Here's how the part is built. I have some questions about the finished solid (model axes, mm). A direction names the side the tool comes from. Round coordinates to 2 decimals unless told otherwise and drop trailing zeros. Loops run counter-clockwise (first coordinate to the right, second up) from the corner with the lowest first, then second, coordinate; pieces in that order, holes last. Notation, with made-up numbers: M -21.75,67.25 L -3.75,67.25 A9 cw -3.75,71.25 Z; hole C -26.5,22.25 d4. An arc over 180 degrees is marked long. Use a Markdown table: item, result.
```python
from build123d import *

# Parameters (mm, degrees)
SKETCH2_R           = 4
BOSS_EXTRUDE1_DEPTH = 25
CUT_EXTRUDE1_DEPTH  = 7
SKETCH6_W           = 0.80480735
SKETCH6_H           = 0.88864145
SKETCH6_W_2         = 0.905408268
BOSS_EXTRUDE2_DEPTH = 5
SKETCH7_R           = 0.3
CUT_EXTRUDE2_DEPTH  = 5


with BuildPart() as part:
    # Sketch2 → Boss-Extrude1 (new body)
    with BuildSketch(Plane(origin=(0, 0, 0), x_dir=(1, 0, 0), z_dir=(0, 1, 0))):
        with Locations(Location((0, 0, 0), (0, 0, 270))):
            Circle(SKETCH2_R)
    extrude(amount=BOSS_EXTRUDE1_DEPTH)

    # Sketch3 → Cut-Extrude1 (cut)
    with BuildSketch(Plane.XZ):
        with BuildLine():
            Line((-4.426440425, 1.819199948), (4.426440425, 1.819199948))
            ThreePointArc((4.426440425, 1.819199948), (0, 4.216961573), (-4.426440425, 1.819199948))
        make_face()
        with BuildLine():
            Line((-4.426440425, -1.819199948), (4.426440425, -1.819199948))
            ThreePointArc((4.426440425, -1.819199948), (0, -4.323632304), (-4.426440425, -1.819199948))
        make_face()
    extrude(amount=-CUT_EXTRUDE1_DEPTH, mode=Mode.SUBTRACT)

    # Sketch6 → Boss-Extrude2 (add)
    with BuildSketch(Plane(origin=(0, 25, 0), x_dir=(1, 0, 0), z_dir=(0, 1, 0))):
        with Locations((-2.39765523, 0)):
            Rectangle(SKETCH6_W, SKETCH6_H)
        with Locations((1.944951096, 0)):
            Rectangle(SKETCH6_W_2, SKETCH6_H)
    extrude(amount=BOSS_EXTRUDE2_DEPTH)

    # Sketch7 → Cut-Extrude2 (cut)
    with BuildSketch(Plane(origin=(0, 0, -0.444320725), x_dir=(-1, 0, 0), z_dir=(0, 0, -1))):
        with Locations((-1.968156059, 29.360387354)):
            Circle(SKETCH7_R)
        with Locations((2.377573757, 29.360387354)):
            Circle(SKETCH7_R)
    extrude(amount=-CUT_EXTRUDE2_DEPTH, mode=Mode.SUBTRACT)


solid = part.part
```
Q1. For faces 5 (the flat face through (2, 27, 0.444)), 6 (the flat face through (2, 27, -0.444)), 7 (the flat face through (0, 3, -1.819)), 8 (the flat face through (0, 7, 3)), which set-ups out of +Z, -Z, +X, -X, +Y, -Y let a thin tool reach every point of the face, with its end or its side?
Return value:
| item | result |
|---|---|
| face 5 | +Z, +X, -X, +Y |
| face 6 | -Z, +X, -X, +Y |
| face 7 | -Z, +X, -X, -Y |
| face 8 | +Z, +X, -X, -Y |
Q2. We'd pull the mould along X, two halves only. Please class faces 1 (the flat face through (1.492, 27, 0)), 2 (the cylindrical face through (0, 15, -4)), 3 (the flat face through (-2.4, 27.5, 0.444)), 4 (the flat face through (-1.995, 27, 0)): pulls with the +X half, pulls with the -X half, needs draft (parallel to the pull), parting line crosses it, or undercut.
Return value:
| item | result |
|---|---|
| face 1 | undercut |
| face 2 | parting line crosses it |
| face 3 | needs draft |
| face 4 | undercut |
Q3. Imagine slicing it at D-D, the plane z = 3. Please give me the cut outline in (x, y), then the cut area to 3 significant figures.
Return value:
| item | result |
|---|---|
| outline | M -2.65,7 L 2.65,7 L 2.65,25 L -2.65,25 Z |
| area | 95.2 mm^2 |
Q4. Imagine slicing it at B-B, the plane z = 0. Please give me the cut outline in (x, y), then the cut area to 3 significant figures.
Return value:
| item | result |
|---|---|
| outline | M -4,0 L 4,0 L 4,25 L 2.4,25 L 2.4,30 L 1.49,30 L 1.49,25 L -2,25 L -2,30 L -2.8,30 L -2.8,25 L -4,25 Z; hole C -2.38,29.36 d0.6; hole C 1.97,29.36 d0.6 |
| area | 208 mm^2 |
Q5. Will these pins go through, and if not, where does the flat tip stop? P1, Ø0.7, axis at y = 27.5, z = 0, coming from the -X side; P2, Ø1.7, axis at x = -1.5, z = -2.5, coming from the -Y side; P3, Ø2, axis at x = 1, z = -2.5, coming from the +Y side; P4, Ø1, axis at x = 3, y = 16.5, coming from the +Z side.
Return value:
| item | result |
|---|---|
| P1 | stops at x = -2.8 |
| P2 | stops at y = 0 |
| P3 | stops at y = 25 |
| P4 | stops at z = 3.12 |
Q6. I need wall thicknesses on line 1 (Y direction, x = 2.25, z = 3); line 2 (Y direction, x = -0.25, z = 0.75); line 3 (X direction, y = 14.25, z = -3). Which ranges of each line are inside material? Lowest first, please. Write a range as from..to.
Return value:
| item | result |
|---|---|
| line 1 | y = 7..25 |
| line 2 | y = 0..25 |
| line 3 | x = -2.65..2.65 |
Q7. Imagine slicing it at A-A, the plane x = 0. Please give me the cut outline in (y, z).
Return value:
| item | result |
|---|---|
| outline | M 0,-1.82 L 7,-1.82 L 7,-4 L 25,-4 L 25,4 L 7,4 L 7,1.82 L 0,1.82 Z |
Q8. Imagine slicing it at C-C, the plane y = 21.25. Please give me the cut outline in (x, z), then the cut area to 3 significant figures.
Return value:
| item | result |
|---|---|
| outline | C 0,0 d8 |
| area | 50.3 mm^2 |
